```python
from build123d import *

# Parameters (mm, degrees)
F0_R     = 11.1
F1_DEPTH = 7
F2_DEPTH = 9


with BuildPart() as f1:
    # F0 (on Top) → F1 (new body)
    with BuildSketch(Plane.XY):
        with BuildLine():
            ThreePointArc((-26.341428, -16.80438), (-16.590351, -18.23282), (-12.994606, -27.40858))
            ThreePointArc((-12.994606, -27.40858), (2.114536, -45.016492), (16.414367, -26.745214))
            ThreePointArc((16.414367, -26.745214), (17.842807, -16.994137), (27.018567, -13.398392))
            ThreePointArc((27.018567, -13.398392), (44.626479, 1.71075), (26.355201, 16.010581))
            ThreePointArc((26.355201, 16.010581), (16.604124, 17.439021), (13.008379, 26.614781))
            ThreePointArc((13.008379, 26.614781), (-2.100763, 44.222693), (-16.400594, 25.951415))
            ThreePointArc((-16.400594, 25.951415), (-17.829034, 16.200338), (-27.004794, 12.604593))
            ThreePointArc((-27.004794, 12.604593), (-44.612706, -2.504549), (-26.341428, -16.80438))
        make_face()
        Circle(F0_R, mode=Mode.SUBTRACT)
    extrude(amount=F1_DEPTH)


with BuildPart() as f2:
    # F0 (on Top) → F2 (new body)
    with BuildSketch(Plane.XY):
        with BuildLine():
            ThreePointArc((-20.216963, 24.70624), (-20.869737, 18.8064), (-26.36112, 16.552751))
            ThreePointArc((-26.36112, 16.552751), (-48.605531, -2.812407), (-25.096253, -20.620749))
            ThreePointArc((-25.096253, -20.620749), (-19.196413, -21.273523), (-16.942764, -26.764906))
            ThreePointArc((-16.942764, -26.764906), (3.243662, -48.963558), (19.770673, -23.920997))
            ThreePointArc((19.770673, -23.920997), (21.425083, -18.978612), (26.374893, -17.34655))
            ThreePointArc((26.374893, -17.34655), (48.573545, 2.839876), (23.530984, 19.366887))
            ThreePointArc((23.530984, 19.366887), (18.588599, 21.021297), (16.956537, 25.971107))
            ThreePointArc((16.956537, 25.971107), (-2.408621, 48.215518), (-20.216963, 24.70624))
        make_face()
        with BuildLine():
            ThreePointArc((16.414367, -26.745214), (2.114536, -45.016492), (-12.994606, -27.40858))
            ThreePointArc((-12.994606, -27.40858), (-16.590351, -18.23282), (-26.341428, -16.80438))
            ThreePointArc((-26.341428, -16.80438), (-44.612706, -2.504549), (-27.004794, 12.604593))
            ThreePointArc((-27.004794, 12.604593), (-17.829034, 16.200338), (-16.400594, 25.951415))
            ThreePointArc((-16.400594, 25.951415), (-2.100763, 44.222693), (13.008379, 26.614781))
            ThreePointArc((13.008379, 26.614781), (16.604124, 17.439021), (26.355201, 16.010581))
            ThreePointArc((26.355201, 16.010581), (44.626479, 1.71075), (27.018567, -13.398392))
            ThreePointArc((27.018567, -13.398392), (17.842807, -16.994137), (16.414367, -26.745214))
        make_face(mode=Mode.SUBTRACT)
        with BuildLine():
            ThreePointArc((-26.341428, -16.80438), (-16.590351, -18.23282), (-12.994606, -27.40858))
            ThreePointArc((-12.994606, -27.40858), (2.114536, -45.016492), (16.414367, -26.745214))
            ThreePointArc((16.414367, -26.745214), (17.842807, -16.994137), (27.018567, -13.398392))
            ThreePointArc((27.018567, -13.398392), (44.626479, 1.71075), (26.355201, 16.010581))
            ThreePointArc((26.355201, 16.010581), (16.604124, 17.439021), (13.008379, 26.614781))
            ThreePointArc((13.008379, 26.614781), (-2.100763, 44.222693), (-16.400594, 25.951415))
            ThreePointArc((-16.400594, 25.951415), (-17.829034, 16.200338), (-27.004794, 12.604593))
            ThreePointArc((-27.004794, 12.604593), (-44.612706, -2.504549), (-26.341428, -16.80438))
        make_face()
        Circle(F0_R, mode=Mode.SUBTRACT)
        Circle(F0_R)
    extrude(amount=F2_DEPTH)

    # F3: cut F1
    add(f1.part, mode=Mode.SUBTRACT)


solid = f2.part
```
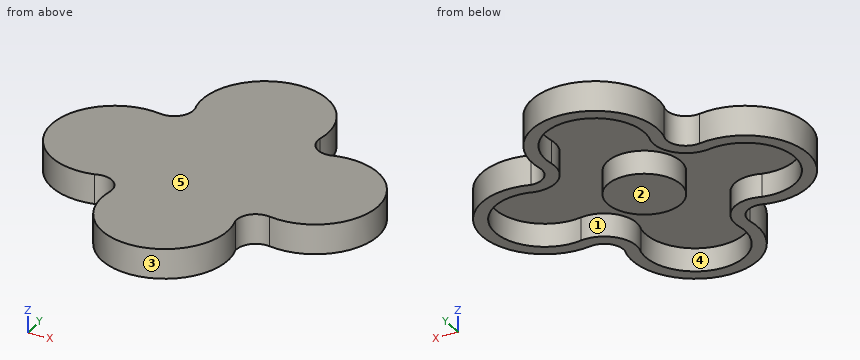
Check sheet for the modelled part. Datum: model origin and axes. Units: mm. Face numbers are marked on the shaded views. A direction names the side the tool comes from. Give positions to 0.01 mm unless a question says otherwise; leave off trailing zeros. Loops run counter-clockwise (first coordinate to the right, second up) from the corner with the lowest first, then second, coordinate; pieces in that order, holes last. Notation, with made-up numbers: (49, 63.5) - (98, 63.5) arc R12 cw to (98, 68.5) - close; hole circle Ø2 at (32.25, -32.75). An arc over 180 degrees is marked (long way). One line per question, with ' | ' between items. Start each with the question number.
1. Draft check along X on the marked faces 3, 4 and 5. Enter one of: released by +X, released by -X, zero draft, split by the parting line, or undercut.
2. Cross-section at D-D, the plane x = 34. Enter the section's corners in (y, z).
3. Gauge pin test, flat ends, axial feed: pin 1 Ø1.5 at (x, y) = (22.5, -26) entering from -Z; pin 2 Ø2 at (y, z) = (-29, 1) entering from +X; pin 3 Ø1.5 at (y, z) = (29, 6.5) entering from -X; pin 4 Ø1.5 at (y, z) = (3.5, 2) entering from -X. Record the tip position at first contact, or that the pin passes through.
4. Cross-section at A-A, the plane z = 3.5. Enter the section's corners in (x, y), plus the area to 3 significant figures.
5. Cross-section at B-B, the plane y = 32.5. Enter the section's corners in (x, z), plus the area to 3 significant figures.
6. Material ranges on line 1 along Y through (x, z) = (3.5, 4); line 2 along X through (y, z) = (4, 5.75); line 3 along Y through (x, z) = (-0.5, 1), recorded low to high. Write a range as [from, to].
7. Cross-section at C-C, the plane x = 0. Enter the section's corners in (y, z).
8. Set-up check for the marked faces 1 and 2: record each of +Z, -Z, +X, -X, +Y, -Y from which the full face is reachable in a straight line by a thin tool's end or side.
Check result:
1) face 3: split by the parting line | face 4: undercut | face 5: zero draft
2) outline: (-17.12, 0) - (-12.98, 0) - (-12.98, 7) - (15.72, 7) - (15.72, 0) - (19.86, 0) - (19.86, 9) - (-17.12, 9) - close
3) pin 1: passes through | pin 2: stops at x = 20.78 | pin 3: stops at x = -20.76 | pin 4: stops at x = -47.97
4) outline: (-26.36, 16.55) arc R19 ccw (long way) to (-25.1, -20.62) arc R5.82 cw to (-16.94, -26.76) arc R19 ccw (long way) to (19.77, -23.92) arc R5.82 cw to (26.37, -17.35) arc R19 ccw (long way) to (23.53, 19.37) arc R5.82 cw to (16.96, 25.97) arc R19 ccw (long way) to (-20.22, 24.71) arc R5.82 cw to start; circle Ø22.2 at (0, 0); hole (-27, 12.6) arc R15 ccw (long way) to (-26.34, -16.8) arc R9.82 cw to (-12.99, -27.41) arc R15 ccw (long way) to (16.41, -26.75) arc R9.82 cw to (27.02, -13.4) arc R15 ccw (long way) to (26.36, 16.01) arc R9.82 cw to (13.01, 26.61) arc R15 ccw (long way) to (-16.4, 25.95) arc R9.82 cw to start | area: 1,620 mm2
5) outline: (-20.48, 0) - (-16.4, 0) - (-16.4, 7) - (12.88, 7) - (12.88, 0) - (16.95, 0) - (16.95, 9) - (-20.48, 9) - close | area: 132 mm2
6) line 1: y = [-48.94, -44.92], [-10.53, 10.53], [43.27, 47.48] | line 2: x = [-47.59, -43.29], [-10.35, 10.35], [44.4, 48.45] | line 3: y = [-48.88, -44.85], [-11.09, 11.09], [44.17, 48.18]
7) outline: (-48.94, 0) - (-44.91, 0) - (-44.91, 7) - (-11.1, 7) - (-11.1, 0) - (11.1, 0) - (11.1, 7) - (44.12, 7) - (44.12, 0) - (48.14, 0) - (48.14, 9) - (-48.94, 9) - close
8) face 1: -Z | face 2: -Z, +X, -X, +Y, -Y
